Read the model definition and answer for the solid it produces. Units are mm, in the model's axes. A direction names the side the tool comes from. Round coordinates to 2 decimals unless told otherwise and drop trailing zeros. Write each loop counter-clockwise with the first axis right and the second up, starting at its lowest first coordinate (ties: lowest second). Pieces come first, ordered by that corner, then holes. Notation, with made-up numbers: (71.25, 84) - (113.25, 84) arc R22 ccw to (113.25, 118) - close; hole circle Ø8 at (87, 77.25). An arc over 180 degrees is marked (long way). Use one line per item in the form item = value. Start each with the question number.
1) The part is cut by section C-C, the plane z = 9.75. Give the vertices of the cut face in (x, y), plus the area to 3 significant figures.
2) For a pull along X with two mould halves and no side action, classify faces 3 (the face through (-4.05, 0, 6)), 4 (the face through (-2, 0, 0)), 5 (the face through (3.25, 0, 3)), 6 (the face through (-1.65, -2.8, 5.02)) as released by +X, released by -X, zero draft, split by the parting line, or undercut.
3) The part is cut by section B-B, the plane x = -1.5. Give the vertices of the cut face in (y, z).
4) Consider line 1 along X through (y, z) = (0, 0.6); line 2 along Z through (x, y) = (-1.75, 0.5). Determine where each line is inside the solid, lowest interval first. Write a range as from..to.
5) The part is cut by section A-A, the plane y = 0. Give the vertices of the cut face in (x, z).
6) The part is cut by section D-D, the plane y = -2.5. Give the vertices of the cut face in (x, z), plus the area to 3 significant figures.
7) Each of these flat-tipped pins is pushed along its axis until it touches: pin 1 (3 mm diameter, centred on x = 1.5, y = 0, fed in from +Z); pin 2 (4 mm diameter, centred on x = 3, z = 5, fed in from -Y); pin 3 (1 mm diameter, centred on x = -1, y = 3, fed in from +Z); pin 4 (1.9 mm diameter, centred on y = 0.5, z = 5, fed in from +X). Where does it stop, or does it pass through?
8) For faces 1 (the face through (-1, 4.05, 5)), 2 (the face through (-1.6, 2.83, 5.02)), determine the directions among +Z, -Z, +X, -X, +Y, -Y from which every point of the face is accessible in a straight line to the end or side of a thin tool.
from build123d import *

# Parameters (mm, degrees)
SKETCH_W             = 8.1
SKETCH_H             = 8.1
SKETCH_R             = 1.75
PAD_DEPTH            = 12
POCKET_DEPTH         = 10.801
POCKET001_DEPTH      = 4.051
POCKET001_DEPTH_BACK = -4.051


with BuildPart() as part:
    # Sketch → Pad (new body)
    with BuildSketch(Plane.XY):
        Rectangle(SKETCH_W, SKETCH_H)
        Circle(SKETCH_R, mode=Mode.SUBTRACT)
    extrude(amount=PAD_DEPTH)

    # Sketch001 → Pocket (cut, through all)
    with BuildSketch(Plane.XY.offset(1.2)):
        Polygon((0, 3.752777), (-3.25, 1.876388), (-3.25, -1.876388), (0, -3.752777), (3.25, -1.876388), (3.25, 1.876388), align=None)
    extrude(amount=POCKET_DEPTH, mode=Mode.SUBTRACT)

    # Sketch002 → Pocket001 (cut, two sides)
    with BuildSketch(Plane.XZ) as pocket001_sk:
        Polygon((4.05, 12), (-4.05, 12), (4.05, 3.9), align=None)
    extrude(amount=-POCKET001_DEPTH, mode=Mode.SUBTRACT)
    extrude(pocket001_sk.sketch, amount=-POCKET001_DEPTH_BACK, mode=Mode.SUBTRACT)


solid = part.part
Geometry results:
q1.outline = (-4.05, -4.05) - (-1.8, -4.05) - (-1.8, -2.71) - (-3.25, -1.88) - (-3.25, 1.88) - (-1.8, 2.71) - (-1.8, 4.05) - (-4.05, 4.05) - close
q1.area = 11.6 mm2
q2.face_3 = released by -X
q2.face_4 = zero draft
q2.face_5 = undercut
q2.face_6 = undercut
q3.outline = (-4.05, 0) - (-0.9, 0) - (-0.9, 1.2) - (-2.89, 1.2) - (-2.89, 9.45) - (-4.05, 9.45) - close; (0.9, 0) - (4.05, 0) - (4.05, 9.45) - (2.89, 9.45) - (2.89, 1.2) - (0.9, 1.2) - close
q4.line_1 = -4.05..-1.75, 1.75..4.05
q4.line_2 = 0..1.2
q5.outline = (-4.05, 0) - (-1.75, 0) - (-1.75, 1.2) - (-3.25, 1.2) - (-3.25, 11.2) - (-4.05, 12) - close; (1.75, 0) - (4.05, 0) - (4.05, 3.9) - (3.25, 4.7) - (3.25, 1.2) - (1.75, 1.2) - close
q6.outline = (-4.05, 0) - (4.05, 0) - (4.05, 3.9) - (2.17, 5.78) - (2.17, 1.2) - (-2.17, 1.2) - (-2.17, 10.12) - (-4.05, 12) - close
q6.area = 35.1 mm2
q7.pin_1 = 1.2
q7.pin_2 = -4.05
q7.pin_3 = 9.45
q7.pin_4 = 3.9
q8.face_1 = +Z, -Z, +X, -X, +Y
q8.face_2 = +Z
